```python
from build123d import *

# Parameters (mm, degrees)
EXTRUDE_1_DEPTH     = 17
FILLET_1_R          = 5
SKETCH_2_R          = 15
EXTRUDE_2_DEPTH     = 3
SKETCH_4_R          = 5
CUT_EXTRUDE_1_DEPTH = 56
SKETCH_3_R          = 7
EXTRUDE_3_DEPTH     = 38
FILLET_2_R          = 10
CHAMFER_1_SIZE      = 1


with BuildPart() as part:
    # 草图1 → 凸台-拉伸1 (new, symmetric)
    with BuildSketch(Plane(origin=(0, 0, 0), x_dir=(1, 0, 0), z_dir=(0, 1, 0))):
        Polygon((20, -87.093671679), (35, -87.093671679), (35, 119.906328321), (-35, 119.906328321), (-35, -87.093671679), (-20, -87.093671679), (-20, 82.906328321), (20, 82.906328321), align=None)
    extrude(amount=EXTRUDE_1_DEPTH, both=True)

    # 圆角1
    fillet_1_edges = [part.edges().sort_by_distance(p)[0] for p in [
        (-35, 0, -119.906328321),
        (35, 0, -119.906328321),
        (20, 0, -82.906328321),
        (-20, 0, -82.906328321),
    ]]
    fillet(fillet_1_edges, radius=FILLET_1_R)

    # 草图2 → 凸台-拉伸2 (add)
    with BuildSketch(Plane(origin=(0, 0, -119.906328321), x_dir=(-1, 0, 0), z_dir=(0, 0, -1))):
        with Locations(Location((0, 0, 0), (0, 0, 180))):
            Circle(SKETCH_2_R)
    extrude(amount=EXTRUDE_2_DEPTH)

    # 草图4 → 切除-拉伸1 (cut, symmetric)
    with BuildSketch(Plane(origin=(0, 0, 0), x_dir=(0, 0, -1), z_dir=(1, 0, 0))):
        with Locations((-67.093671679, 0)):
            Circle(SKETCH_4_R)
    extrude(amount=CUT_EXTRUDE_1_DEPTH, both=True, mode=Mode.SUBTRACT)

    # 草图3 → 凸台-拉伸3 (add)
    with BuildSketch(Plane(origin=(0, 0, -122.906328321), x_dir=(-1, 0, 0), z_dir=(0, 0, -1))):
        Circle(SKETCH_3_R)
    extrude(amount=EXTRUDE_3_DEPTH)

    # 圆角2
    fillet_2_edges = [part.edges().sort_by_distance(p)[0] for p in [
        (-27.5, -17, 87.093671679),
        (27.5, 17, 87.093671679),
        (-27.5, 17, 87.093671679),
        (27.5, -17, 87.093671679),
    ]]
    fillet(fillet_2_edges, radius=FILLET_2_R)

    # 倒角1
    chamfer_1_edges = [part.edges().sort_by_distance(p)[0] for p in [
        (7, 0, -160.906328321),
    ]]
    chamfer(chamfer_1_edges, length=CHAMFER_1_SIZE)


solid = part.part
```
Work out the finished part from the listing and answer in its coordinate system (mm). A direction names the side the tool comes from. Coordinates: 2 decimals unless noted, no trailing zeros. Order: outer loops, then holes, each group sorted by start corner. A loop starts at its lowest first (then second) coordinate and runs counter-clockwise, first axis right, second up. Notation, with made-up numbers: M 83.5,-3.5 L 101.5,-3.5 A4 ccw 101.5,1.5 Z; hole C -23.75,25.25 d3. An arc over 180 degrees is marked long. Use CSV: the item, a comma, the result in double quotes.
1) Section D-D on x = -9.5 is taken. Write down the section's boundary in (y, z), plus the area to 3 significant figures.
Worked out:
outline,"M -17,-119.91 L -11.61,-119.91 L -11.61,-122.91 L 11.61,-122.91 L 11.61,-119.91 L 17,-119.91 L 17,-82.91 L -17,-82.91 Z"
area,"1,330 mm^2"
2) Section A-A on z = 28.5 is taken. Write down the section's boundary in (x, y), plus the area to 3 significant figures.
Worked out:
outline,"M -35,-17 L -20,-17 L -20,17 L -35,17 Z; M 20,-17 L 35,-17 L 35,17 L 20,17 Z"
area,"1,020 mm^2"
3) Consider line 1 (X direction, y = -1, z = 29); line 2 (Z direction, x = -4, y = -10); line 3 (Z direction, x = 12, y = -13). Determine where each line is inside the solid, lowest interval first. Write a range as [from, to].
Worked out:
line 1,"x = [-35, -20], [20, 35]"
line 2,"z = [-122.91, -82.91]"
line 3,"z = [-119.91, -82.91]"
4) Section C-C on x = 0 is taken. Write down the section's boundary in (y, z), plus the area to 3 significant figures.
Worked out:
outline,"M -17,-119.91 L -15,-119.91 L -15,-122.91 L -7,-122.91 L -7,-159.91 L -6,-160.91 L 6,-160.91 L 7,-159.91 L 7,-122.91 L 15,-122.91 L 15,-119.91 L 17,-119.91 L 17,-82.91 L -17,-82.91 Z"
area,"1,880 mm^2"
5) Determine the mould class of faces 4 (the face through (27.6, 0.22, 72.09)), 5 (the face through (-27.395, 14.148, 84.087)), 6 (the face through (-20, 0, 6)) for opening direction Y: released by +Y, released by -Y, zero draft, split by the parting line, or undercut.
Worked out:
face 4,"undercut"
face 5,"released by +Y"
face 6,"zero draft"
6) Flat-ended cylindrical pins translate along their axes: pin 1 Ø1.5 at (x, y) = (-26, -3.5) entering from -Z; pin 2 Ø5 at (x, z) = (7, -130.5) entering from +Y. Find the tip coordinate at first contact, or state that the pin passes through.
Worked out:
pin 1,"stops at z = -119.91"
pin 2,"stops at y = 5.36"
7) For faces 1 (the face through (8.06, -12.65, -121.39)), 2 (the face through (-27.4, 0.22, 72.09)), 3 (the face through (18.574, -0.238, -81.403)), determine the directions among +Z, -Z, +X, -X, +Y, -Y from which every point of the face is accessible in a straight line to the end or side of a thin tool.
Worked out:
face 1,"-Z"
face 2,"+X, -X"
face 3,"+Z, +Y, -Y"
8) Section B-B on y = 0 is taken. Count the separate pieces of the cut face and the enclosed holes in it, plus the area to 3 significant figures.
Worked out:
separate pieces,"3"
enclosed holes,"0"
area,"8,010 mm^2"
